Read the model definition and answer for the solid it produces. Units are mm, in the model's axes. A direction names the side the tool comes from. Give positions to 0.01 mm unless a question says otherwise; leave off trailing zeros. Loops run counter-clockwise (first coordinate to the right, second up) from the corner with the lowest first, then second, coordinate; pieces in that order, holes last. Notation, with made-up numbers: (0, 64.25) - (13, 64.25) arc R7 cw to (13, 68.25) - close; hole circle Ø11 at (-40, 23). An arc over 180 degrees is marked (long way). Use a Markdown table: item, result. Add a question column.
Item 1: Each of these flat-tipped pins is pushed along its axis until it touches: P1, Ø1.3, axis at y = -1, z = 19, coming from the -X side; P2, Ø1.3, axis at y = 4, z = 19.5, coming from the +X side; P3, Ø1.5, axis at x = -1, y = -2, coming from the -Z side; P4, Ø2, axis at x = 1, z = 34.5, coming from the -Y side. Where does it stop, or does it pass through?
Item 2: For a pull along X with two mould halves and no side action, classify faces 4 (the face through (-2.5, 4, 25)), 5 (the face through (0, 5, 7.5)), 6 (the face through (-2.5, -1, 25)) as +X half, -X half, draft (parallel to the pull), parting line (faces both ways), or undercut.
Item 3: A cutting plane is placed at B-B (z = 17). Determine the outline of the cut face in (x, y).
Item 4: A cutting plane is placed at A-A (x = 0). Determine the outline of the cut face in (y, z).
Item 5: Consider probe 1 along X at (y, z) = (2.5, 4.5); probe 2 along X at (y, z) = (3.75, 37.5); probe 3 along Z at (x, y) = (-1.6, 6.5). Determine where each line is inside the solid, lowest interval first. Write a range as [from, to].
Item 6: Which of the six approach directions +Z, -Z, +X, -X, +Y, -Y give full straight-line access (tool end or side, diameter ignored) to faces 1 (the face through (0, 0, 50)), 2 (the face through (0, -2.7, 7.5)), 3 (the face through (2.5, 4, 25))?
Item 7: A cutting plane is placed at C-C (y = 7.5). Determine the outline of the cut face in (x, z), plus the area to 3 significant figures.
Autodesk Inventor part; units mm, degrees
ref_plane "YZ Plane" through (0, 0, 0) normal (1, 0, 0) x (0, 1, 0)
ref_plane "XZ Plane" through (0, 0, 0) normal (0, 1, 0) x (-1, 0, 0)
ref_plane "XY Plane" through (0, 0, 0) normal (0, 0, 1) x (1, 0, 0)
sketch "Эскиз4" plane through (0, 0, 0) normal (0, 0, 1) x (1, 0, 0)
  circle A0 centre (0, 0) radius 3
  dimension "d8" = 6
extrude "Выдавливание3" add sketch "Эскиз4" along normal blind 50
sketch "Эскиз5" plane through (0, 0, 0) normal (0, 1, 0) x (-1, 0, 0)
  line L0 (0, 0) -> (0, 25)
  line L1 (-2.5, 42.5) -> (2.5, 42.5)
  line L2 (2.5, 42.5) -> (2.5, 7.5)
  line L3 (2.5, 7.5) -> (-2.5, 7.5)
  line L4 (-2.5, 7.5) -> (-2.5, 42.5)
  line L5 (-2.5, 42.5) -> (2.5, 7.5) construction
  line L6 (2.5, 42.5) -> (-2.5, 7.5) construction
  dimension "d11" = 25
  dimension "d12" = 5
  dimension "d13" = 35
extrude "Выдавливание4" cut sketch "Эскиз5" against normal mid plane 50
sketch "Эскиз6" plane through (0, 0, 42.5) normal (0, 0, -1) x (-1, 0, 0)
  point P0 (0, 0)
sketch "Эскиз7" plane through (0, 0, 7.5) normal (0, 0, 1) x (1, 0, 0)
  circle A0 centre (0, 0) radius 3
  line L0 (0, 0) -> (0, 6) construction
  arc A1 (2.5, 1.6583) -> (-2.5, 1.6583) centre (0, 0) ccw
  line L1 (2.5, 0) -> (2.5, 6)
  line L2 (-2.5, 6) -> (-2.5, 0)
  arc A2 (-2.5, 0) -> (2.5, 0) centre (0, 0) ccw
  arc A3 (2.5, 6) -> (-2.5, 6) centre (0, 6) ccw
  point P0 (1, 1)
  point P1 (0, 3)
  dimension "d16" = 3
  dimension "d17" = 5
extrude "Выдавливание5" add sketch "Эскиз7" along normal blind 35 contours L1 A2 L2 A0 | A0 L2 A3 L1 picked at (0, 1)
properties part number "ведущий вал"
Geometry says:
| question | item | result |
|---|---|---|
| 1 | P1 | x = -2.98 |
| 1 | P2 | x = 2.5 |
| 1 | P3 | z = 0 |
| 1 | P4 | y = -2.5 |
| 2 | face 4 | -X half |
| 2 | face 5 | draft |
| 2 | face 6 | undercut |
| 3 | outline | (-2.5, -1.66) - (-2.5, 0) arc R2.5 ccw to (2.5, 0) - (2.5, -1.66) arc R3 ccw to (2.5, 1.66) - (2.5, 6) arc R2.5 ccw to (-2.5, 6) - (-2.5, 1.66) arc R3 ccw to start |
| 4 | outline | (-3, 0) - (3, 0) - (3, 7.5) - (8.5, 7.5) - (8.5, 42.5) - (3, 42.5) - (3, 50) - (-3, 50) - (-3, 42.5) - (-2.5, 42.5) - (-2.5, 7.5) - (-3, 7.5) - close |
| 5 | probe 1 | [-1.66, 1.66] |
| 5 | probe 2 | [-2.5, 2.5] |
| 5 | probe 3 | [7.5, 42.5] |
| 6 | face 1 | +Z, +X, -X, +Y, -Y |
| 6 | face 2 | -Y |
| 6 | face 3 | +Z, -Z, +X, +Y |
| 7 | outline | (-2, 7.5) - (2, 7.5) - (2, 42.5) - (-2, 42.5) - close |
| 7 | area | 140 mm² |
